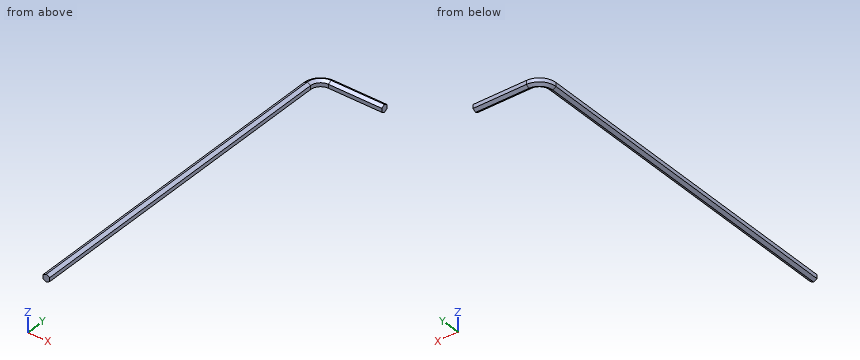
from build123d import *


with BuildPart() as part:
    # 6mm: sweep along a path in Sketch1
    with BuildLine(Plane.XY) as f_6mm_path:
        Line((0, 0), (-12, 0))
        ThreePointArc((-12, 0), (-14.121320344, -0.878679656), (-15, -3))
        Line((-15, -3), (-15, -78))
    # Sketch 6m → 6mm (sweep)
    with BuildSketch(Plane(origin=(0, 0, 0), x_dir=(0, 0, -1), z_dir=(1, 0, 0))):
        Polygon((-0.866025404, 0), (-0.433012702, -0.75), (0.433012702, -0.75), (0.866025404, 0), (0.433012702, 0.75), (-0.433012702, 0.75), align=None)
    sweep(path=f_6mm_path.line)


solid = part.part
Read the model definition and answer for the solid it produces. Units are mm, in the model's axes. Round coordinates to 2 decimals unless told otherwise and drop trailing zeros. Order: outer loops, then holes, each group sorted by start corner. A loop starts at its lowest first (then second) coordinate and runs counter-clockwise, first axis right, second up. Notation, with made-up numbers: (56.25, -6.5) - (87.25, -6.5) arc R16 cw to (87.25, 15.5) - close; hole circle Ø5 at (65.25, 4). An arc over 180 degrees is marked (long way). Use one line per item in the form item = value. Start each with the question number.
(1) A flat-ended cylindrical pin translates along its axis: pin 1 Ø0.7 at (y, z) = (-35, 0) entering from +X. Find the tip coordinate at first contact, or state that the pin passes through.
(2) The part is cut by section A-A (z = 0). Give the vertices of the cut face in (x, y), then the cut area to 3 significant figures.
(3) The part is cut by section C-C (y = -8.5). Give the vertices of the cut face in (x, z).
(4) Find the intervals of material crossed by line 1 along Y through (x, z) = (-7.75, -0.2); line 2 along X through (y, z) = (-41, 0.05); line 3 along X through (y, z) = (-21, -0.55), in increasing order. Write a range as from..to.
(5) The part is cut by section B-B (x = -4.5). Give the vertices of the cut face in (y, z), then the cut area to 3 significant figures.
Checked values:
q1.pin_1 = -14.25
q2.outline = (-15.75, -78) - (-14.25, -78) - (-14.25, -3) arc R2.25 cw to (-12, -0.75) - (0, -0.75) - (0, 0.75) - (-12, 0.75) arc R3.75 ccw to (-15.75, -3) - close
q2.area = 138 mm^2
q3.outline = (-15.75, -0.43) - (-15, -0.87) - (-14.25, -0.43) - (-14.25, 0.43) - (-15, 0.87) - (-15.75, 0.43) - close
q4.line_1 = -0.75..0.75
q4.line_2 = -15.75..-14.25
q4.line_3 = -15.55..-14.45
q5.outline = (-0.75, -0.43) - (0, -0.87) - (0.75, -0.43) - (0.75, 0.43) - (0, 0.87) - (-0.75, 0.43) - close
q5.area = 1.95 mm^2
